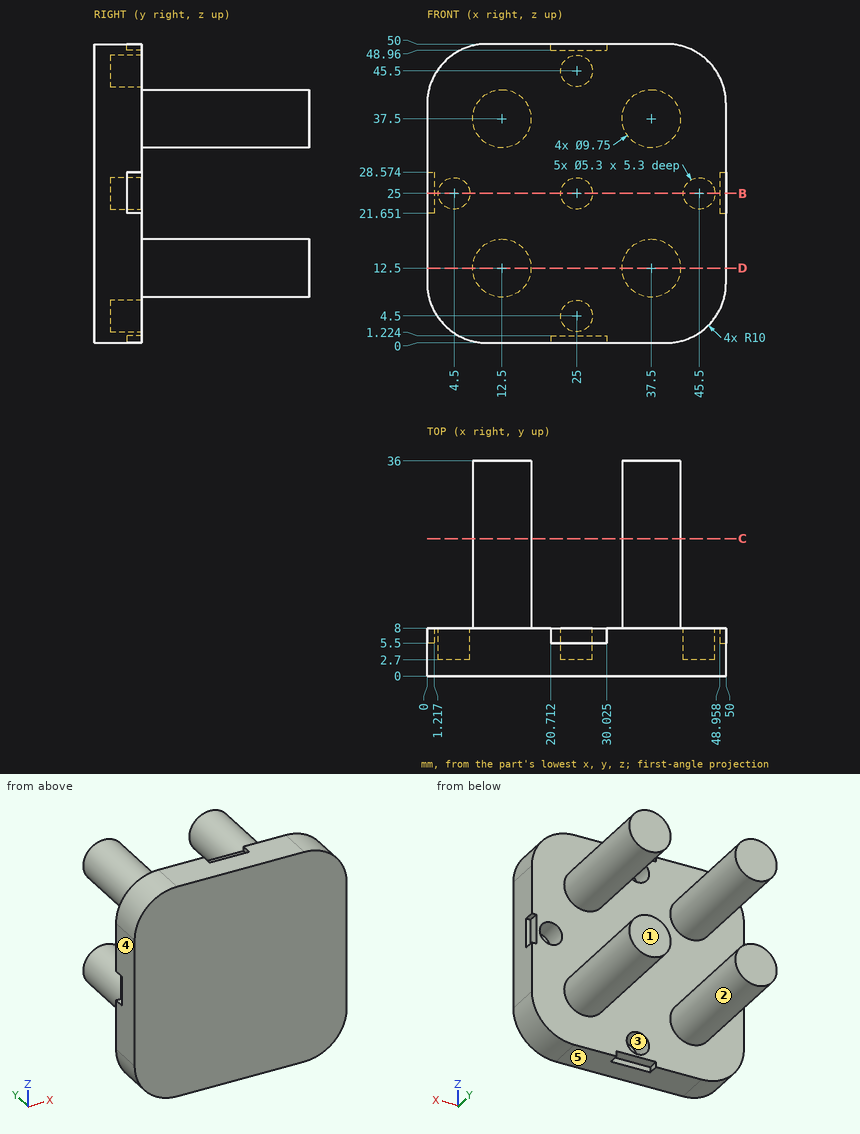
Can you work these out from the drawing? Everything is in mm from the part's minimum corner. A direction names the side the tool comes from. Coordinates: 2 decimals unless noted, no trailing zeros. Loops run counter-clockwise (first coordinate to the right, second up) from the corner with the lowest first, then second, coordinate; pieces in that order, holes last.
1) For pin 1 (3 mm diameter, centred on x = 18, y = 27, fed in from -Z) (1 decimal); pin 2 (0.6 mm diameter, centred on y = 7, z = 0.5, fed in from -X); pin 3 (1.2 mm diameter, centred on y = 7, z = 26, fed in from +X), each with a flat end and sliding along its axis, tell me the tip position at first contact or that it passes through.
2) I need wall thicknesses on probe 1 along X at (y, z) = (6.55, 25); probe 2 along X at (y, z) = (5.2, 25); probe 3 along Y at (x, z) = (27.5, 14). Which ranges of each line are inside material? Lowest first, please.
3) Imagine slicing it at D-D on z = 12.5. List the corners of the cut face in (x, y) for me (1 decimal).
4) Imagine slicing it at B-B on z = 25. List the corners of the cut face in (x, y) for me, plus the area to 3 significant figures.
5) Thinking about a two-plate mould opening in Z: for the marked faces 3, 4 and 5, which applies, pulls with the +Z half, pulls with the -Z half, needs draft (parallel to the pull), parting line crosses it, or undercut?
6) Imagine slicing it at C-C on y = 23. State how many separate pieces and enclosed holes the cut face has, plus the area to 3 significant figures.
7) Which directions (+Z, -Z, +X, -X, +Y, -Y) give clear straight access to the entire face, cutting with the end or side of a thin tool? Please do the marked faces 1 and 2.
Completed:
1. pin 1: stops at z = 9.7
1. pin 2: stops at x = 6.08
1. pin 3: stops at x = 48.96
2. probe 1: x = 1.22 to 1.85, 7.15 to 22.35, 27.65 to 42.85, 48.15 to 48.96
2. probe 2: x = 0 to 1.85, 7.15 to 22.35, 27.65 to 42.85, 48.15 to 50
2. probe 3: y = 0 to 8
3. outline: (0, 0) - (50, 0) - (50, 8) - (42.4, 8) - (42.4, 36) - (32.6, 36) - (32.6, 8) - (17.4, 8) - (17.4, 36) - (7.6, 36) - (7.6, 8) - (0, 8) - close
4. outline: (0, 0) - (50, 0) - (50, 5.5) - (48.96, 5.5) - (48.96, 8) - (48.15, 8) - (48.15, 2.7) - (42.85, 2.7) - (42.85, 8) - (27.65, 8) - (27.65, 2.7) - (22.35, 2.7) - (22.35, 8) - (7.15, 8) - (7.15, 2.7) - (1.85, 2.7) - (1.85, 8) - (1.22, 8) - (1.22, 5.5) - (0, 5.5) - close
4. area: 310 mm2
5. face 3: undercut
5. face 4: needs draft
5. face 5: pulls with the -Z half
6. separate pieces: 4
6. enclosed holes: 0
6. area: 299 mm2
7. face 1: +Z, -Z, +X, -X, +Y
7. face 2: +Y
